```python
from build123d import *

# Parameters (mm, degrees)
SKETCH2_R           = 75
BOSS_EXTRUDE1_DEPTH = 20
FILLET1_R           = 5
BOSS_EXTRUDE2_DEPTH = 5
CHAMFER4_SIZE       = 2.5
FILLET2_R           = 5
SKETCH7_R           = 10
BOSS_EXTRUDE3_DEPTH = 2.5
CHAMFER5_SIZE       = 2.5
SKETCH8_R           = 5
CUT_EXTRUDE1_DEPTH  = 10


with BuildPart() as part:
    # Sketch2 → Boss-Extrude1 (new body)
    with BuildSketch(Plane(origin=(0, 0, 0), x_dir=(1, 0, 0), z_dir=(0, 1, 0))):
        with Locations(Location((0, 0, 0), (0, 0, 270))):
            Circle(SKETCH2_R)
    extrude(amount=BOSS_EXTRUDE1_DEPTH)

    # Fillet1
    fillet1_edges = [part.edges().sort_by_distance(p)[0] for p in [
        (0, 20, -75),
    ]]
    fillet(fillet1_edges, radius=FILLET1_R)

    # Sketch3 → Boss-Extrude2 (add, symmetric)
    with BuildSketch(Plane.XY):
        with BuildLine():
            Line((-35, 15), (30, 15))
            ThreePointArc((30, 15), (17.428098582, 56.126843631), (14.970645506, 99.06203778))
            ThreePointArc((14.970645506, 99.06203778), (6.012327577, 113.742340307), (-10.849201429, 110.358321696))
            ThreePointArc((-10.849201429, 110.358321696), (-35.460543036, 65.854059614), (-35, 15))
        make_face()
    extrude(amount=BOSS_EXTRUDE2_DEPTH, both=True)

    # Chamfer4
    chamfer4_edges = [part.edges().sort_by_distance(p)[0] for p in [
        (-34.796467261, 68.341174934, -5),
        (16.970295051, 58.803839559, -5),
        (6.012327577, 113.742340307, -5),
        (16.970295051, 58.803839559, 5),
        (6.012327577, 113.742340307, 5),
        (-34.796467261, 68.341174934, 5),
    ]]
    chamfer(chamfer4_edges, length=CHAMFER4_SIZE)

    # Fillet2
    fillet2_edges = [part.edges().sort_by_distance(p)[0] for p in [
        (-4.241511046, 20, 5),
        (-4.241511046, 20, -5),
    ]]
    fillet(fillet2_edges, radius=FILLET2_R)

    # Sketch7 → Boss-Extrude3 (add, symmetric)
    with BuildSketch(Plane.XY.offset(5)):
        with Locations(Location((0, 100, 0), (0, 0, 180))):
            Circle(SKETCH7_R)
    extrude(amount=BOSS_EXTRUDE3_DEPTH, both=True)

    # Chamfer5
    chamfer5_edges = [part.edges().sort_by_distance(p)[0] for p in [
        (10, 100, 7.5),
    ]]
    chamfer(chamfer5_edges, length=CHAMFER5_SIZE - 0.0001)  # a hair under: the kernel refuses the full size

    # Sketch8 → Cut-Extrude1 (cut)
    with BuildSketch(Plane(origin=(0, 0, -5), x_dir=(-1, 0, 0), z_dir=(0, 0, -1))):
        with Locations((0, 100)):
            Circle(SKETCH8_R)
    extrude(amount=-CUT_EXTRUDE1_DEPTH, mode=Mode.SUBTRACT)


solid = part.part
```
Verification items for the finished model (mm, model axes). A direction names the side the tool comes from. Coordinates: 2 decimals unless noted, no trailing zeros. Loops run counter-clockwise (first coordinate to the right, second up) from the corner with the lowest first, then second, coordinate; pieces in that order, holes last. Notation, with made-up numbers: (-32.75, 70) - (21.25, 70) arc R24 ccw to (21.25, 84) - close; hole circle Ø1 at (45.5, 0.5). An arc over 180 degrees is marked (long way). Put each result on its own line as item: value.
Item 1: Draft check along Y on faces 1 (the face through (1, 0, -1)), 2 (the face through (-45.636, 7.395, -59.517)), 3 (the face through (17.06, 58.25, 0.04)), 4 (the face through (-5, 21, 7)). Enter one of: pulls with the +Y half, pulls with the -Y half, needs draft (parallel to the pull), parting line crosses it, or undercut.
Conclusion:
face 1: pulls with the -Y half
face 2: needs draft
face 3: undercut
face 4: undercut
Item 2: Gauge pin test, flat ends, axial feed: pin 1 Ø1.5 at (x, z) = (14, 11.5) entering from +Y; pin 2 Ø16.5 at (x, y) = (-1.5, 99) entering from +Z; pin 3 Ø3 at (x, y) = (-0.5, 98.5) entering from -Z; pin 4 Ø5 at (x, y) = (21, 57.5) entering from +Z. Record the tip position at first contact, or that the pin passes through.
Conclusion:
pin 1: stops at y = 20
pin 2: stops at z = 7.5
pin 3: stops at z = 5
pin 4: passes through
Item 3: Set-up check for faces 5 (the face through (-7, 60, -5)), 6 (the face through (0, 100, 5)), 7 (the face through (0, 100, 7.5)): record each of +Z, -Z, +X, -X, +Y, -Y from which the full face is reachable in a straight line by a thin tool's end or side.
Conclusion:
face 5: -Z, +X, -X, +Y
face 6: -Z
face 7: +Z, +X, -X, +Y
Item 4: Scan lines: line 1 along Y through (x, z) = (0, 1.5); line 2 along Y through (x, z) = (20, -16); line 3 along Z through (x, y) = (0, 39). Record each from-to range of solid material in increasing order.
Conclusion:
line 1: y = 0 to 95, 105 to 115
line 2: y = 0 to 20
line 3: z = -5 to 5
Item 5: Section check B-B (z = 0). Enter the section's corners in (x, y), then the cut area to 3 significant figures.
Conclusion:
outline: (-75, 0) - (75, 0) - (75, 15) arc R5 ccw to (70, 20) - (27.88, 20) arc R180 cw to (14.97, 99.06) arc R15 ccw to (-10.85, 110.36) arc R100 ccw to (-36.23, 20) - (-70, 20) arc R5 ccw to (-75, 15) - close; hole circle Ø10 at (0, 100)
area: 7,460 mm2
